from build123d import *

# Parameters (mm, degrees)
F2_SIZE = 1


with BuildPart() as f1:
    # F0 (on Right) → F1 (revolve)
    with BuildSketch(Plane.YZ):
        Polygon((0, 9.75), (7, 9.75), (7, 11.5), (2, 11.5), (2, 12.5), (0, 12.5), align=None)
    revolve(axis=Axis((0, 5.735075, 0), (0, -1, 0)))

    # F2
    f2_edges = [f1.edges().sort_by_distance(p)[0] for p in [
        (0, 7, -11.5),
    ]]
    chamfer(f2_edges, length=F2_SIZE)


solid = f1.part
Geometry: final body of the model. Coordinates: model frame, mm. A direction names the side the tool comes from. Coordinates: 2 decimals unless noted, no trailing zeros. Write each loop counter-clockwise with the first axis right and the second up, starting at its lowest first coordinate (ties: lowest second). Pieces come first, ordered by that corner, then holes. Notation, with made-up numbers: (46.5, 72.5) - (100.5, 72.5) arc R15 cw to (100.5, 97.5) - close; hole circle Ø2 at (27.25, 6.5). An arc over 180 degrees is marked (long way). Return JSON: item names as keys, results as strings.
Item 1: Line query: L1, parallel to X at y = 2.75, z = 0; L2, parallel to X at y = 1.75, z = 0. Output: solid intervals per line, ascending.
Completed:
{"L1": "x = -11.5 to -9.75, 9.75 to 11.5", "L2": "x = -12.5 to -9.75, 9.75 to 12.5"}
Item 2: Pin query (flat end, axial travel): pin 1 Ø2 at (y, z) = (3.5, 3) entering from -X. Return the tip coordinate at first contact, or that it passes through.
Completed:
{"pin 1": "stops at x = -11.32"}
Item 3: Reachability of faces 4 (the face through (4, 2, -11)), 5 (the face through (-3.755, 0.986, 11.923)) from +Z, -Z, +X, -X, +Y, -Y: full face, straight path, thin tool, end or side. Return the list, or none.
Completed:
{"face 4": "+Y", "face 5": "+Y, -Y"}
Item 4: Pull-direction query (Z, two-part tool) for faces 1 (the face through (-9.667, 3.549, -1.269)), 2 (the face through (8, 7, -6)), 3 (the face through (-11.4, 4, -1.5)); classes: +Z half, -Z half, draft (parallel to the pull), parting line (faces both ways), or undercut.
Completed:
{"face 1": "undercut", "face 2": "draft", "face 3": "parting line"}
Item 5: Section query A-A (x = 0). Output: boundary loops of the cut face in (y, z), and give its area (3 significant figures).
Completed:
{"outline": "(0, -12.5) - (2, -12.5) - (2, -11.5) - (6, -11.5) - (7, -10.5) - (7, -9.75) - (0, -9.75) - close; (0, 9.75) - (7, 9.75) - (7, 10.5) - (6, 11.5) - (2, 11.5) - (2, 12.5) - (0, 12.5) - close", "area": "27.5 mm2"}
Item 6: Section query B-B (z = 0). Output: boundary loops of the cut face in (x, y).
Completed:
{"outline": "(-12.5, 0) - (-9.75, 0) - (-9.75, 7) - (-10.5, 7) - (-11.5, 6) - (-11.5, 2) - (-12.5, 2) - close; (9.75, 0) - (12.5, 0) - (12.5, 2) - (11.5, 2) - (11.5, 6) - (10.5, 7) - (9.75, 7) - close"}
Item 7: Section query C-C (y = 5.5). Output: boundary loops of the cut face in (x, z).
Completed:
{"outline": "circle Ø23 at (0, 0); hole circle Ø19.5 at (0, 0)"}
